CAD build for the part. Positions are in the model's coordinates, mm. A direction names the side the tool comes from. Round coordinates to 2 decimals unless told otherwise and drop trailing zeros. Order: outer loops, then holes, each group sorted by start corner. A loop starts at its lowest first (then second) coordinate and runs counter-clockwise, first axis right, second up. Notation, with made-up numbers: M -30.75,79 L 4.25,79 A27 cw 4.25,101 Z; hole C -34.5,49 d4. An arc over 180 degrees is marked long. Answer as a JSON object with one key per item and string values.
```python
from build123d import *

# Parameters (mm, degrees)
SKETCH_1_W                   = 25
SKETCH_1_H                   = 10
EXTRUDE_1_DEPTH              = 4
SKETCH_2_W                   = 7
SKETCH_2_H                   = 1
CUT_EXTRUDE_1_DEPTH          = 17.5
HOLE_WIZARD_M3_1_D           = 3.4
HOLE_WIZARD_M3_1_CSINK_D     = 6.6
HOLE_WIZARD_M3_1_CSINK_ANGLE = 90
FILLET_1_R                   = 2
CHAMFER_1_SIZE               = 0.4
CUT_EXTRUDE_2_DEPTH          = 0.4


with BuildPart() as part:
    # 草图1 → 凸台-拉伸1 (new body)
    with BuildSketch(Plane.XY):
        Rectangle(SKETCH_1_W, SKETCH_1_H)
    extrude(amount=EXTRUDE_1_DEPTH)

    # 草图2 → 切除-拉伸1 (cut, through all)
    with BuildSketch(Plane(origin=(0, 5, 0), x_dir=(1, 0, 0), z_dir=(0, 1, 0))):
        Rectangle(SKETCH_2_W, SKETCH_2_H)
    extrude(amount=-CUT_EXTRUDE_1_DEPTH, mode=Mode.SUBTRACT)

    # M3 十字槽沉头木螺钉的锥形沉头孔1 (through all)
    with Locations(Plane.XY.offset(4)):
        with Locations((7, 0)):
            hole_wizard_m3_1 = CounterSinkHole(HOLE_WIZARD_M3_1_D / 2, HOLE_WIZARD_M3_1_CSINK_D / 2, counter_sink_angle=HOLE_WIZARD_M3_1_CSINK_ANGLE)

    # 镜向1: M3 十字槽沉头木螺钉的锥形沉头孔1 across plane
    add(hole_wizard_m3_1.mirror(Plane(origin=(0, 0, 0), x_dir=(0, 0, 1), z_dir=(1, 0, 0))), mode=Mode.SUBTRACT)

    # 圆角1
    fillet_1_edges = [part.edges().sort_by_distance(p)[0] for p in [
        (12.5, -5, 2),
        (-12.5, -5, 2),
        (-12.5, 5, 2),
        (12.5, 5, 2),
    ]]
    fillet(fillet_1_edges, radius=FILLET_1_R)

    # 倒角1
    chamfer_1_edges = [part.edges().sort_by_distance(p)[0] for p in [
        (-12.5, 0, 4),
        (0, 5, 4),
        (12.5, 0, 4),
        (0, -5, 4),
        (11.914213562, 4.414213562, 4),
        (11.914213562, -4.414213562, 4),
        (-11.914213562, -4.414213562, 4),
        (-11.914213562, 4.414213562, 4),
    ]]
    chamfer(chamfer_1_edges, length=CHAMFER_1_SIZE)

    # 草图5 → 切除-拉伸2 (cut)
    with BuildSketch(Plane(origin=(0, 0, 0.5), x_dir=(-1, 0, 0), z_dir=(0, 0, -1))):
        Polygon((-3.5, -2.085786438), (-3.5, -3.5), (3.5, 3.5), (3.5, 4.914213562), align=None)
        Polygon((3.5, 0.5), (3.5, 1.914213562), (-3.414213562, -5), (-2, -5), align=None)
        Polygon((-3.5, 0.914213562), (-3.5, -0.5), (2, 5), (0.585786438, 5), align=None)
        Polygon((3.5, -2.5), (3.5, -1.085786438), (-0.414213562, -5), (1, -5), align=None)
        Polygon((-3.5, 3.914213562), (-3.5, 2.5), (-1, 5), (-2.414213562, 5), align=None)
        Polygon((3.5, -5), (3.5, -4.085786438), (2.585786438, -5), align=None)
    extrude(amount=-CUT_EXTRUDE_2_DEPTH, mode=Mode.SUBTRACT)


solid = part.part
```
Item 1: Saw through at B-B on z = 3.35. List the corners of the cut face in (x, y), and give its area (3 significant figures).
Worked answers:
{"outline": "M -12.5,-3 A2 ccw -10.5,-5 L 10.5,-5 A2 ccw 12.5,-3 L 12.5,3 A2 ccw 10.5,5 L -10.5,5 A2 ccw -12.5,3 Z; hole C -7,0 d5.3; hole C 7,0 d5.3", "area": "202 mm2"}
Item 2: Saw through at C-C on y = 0. State how many separate pieces and enclosed holes the cut face has, and give its area (3 significant figures).
Worked answers:
{"separate pieces": "3", "enclosed holes": "0", "area": "62.7 mm2"}
Item 3: Wall check: line 1 along X through (y, z) = (0, 1.4); line 2 along Y through (x, z) = (-7, 1.5); line 3 along Y through (x, z) = (-3.25, 0.6). Give the ranges that are in metal, low to high. Write a range as [from, to].
Worked answers:
{"line 1": "x = [-12.5, -8.7], [-5.3, 5.3], [8.7, 12.5]", "line 2": "y = [-5, -1.7], [1.7, 5]", "line 3": "y = [-4.34, -2.75], [-1.34, 0.25], [1.66, 3.25], [4.66, 5]"}
Item 4: Drop a flat-ended pin along its axis: pin 1 Ø3 at (x, y) = (1.5, 4) entering from -Z. Give the stop position or say it passes through.
Worked answers:
{"pin 1": "stops at z = 0.5"}
Item 5: 3-axis set-ups, long thin cutter, end or side, ignore diameter. For faces 1 (the flat face through (-2.2, -3.8, 0.7)), 2 (the flat face through (-1, -3, 0.5)), 3 (the flat face through (-9, 0, 0)): which of +Z, -Z, +X, -X, +Y, -Y reach the whole face in a straight line?
Worked answers:
{"face 1": "-Z", "face 2": "-Z, +Y, -Y", "face 3": "-Z, +X, -X, +Y, -Y"}
Item 6: Saw through at D-D on z = 1.75. List the corners of the cut face in (x, y), and give its area (3 significant figures).
Worked answers:
{"outline": "M -12.5,-3 A2 ccw -10.5,-5 L 10.5,-5 A2 ccw 12.5,-3 L 12.5,3 A2 ccw 10.5,5 L -10.5,5 A2 ccw -12.5,3 Z; hole C -7,0 d3.4; hole C 7,0 d3.4", "area": "228 mm2"}
Item 7: Two-plate mould, pull along Y, no slides. Class faces 4 (the flat face through (-0.049, 1.463, 0.697)), 5 (the cylindrical face through (11.93, 4.4, 1.83)), 6 (the flat face through (9, 0, 0)), 7 (the cylindrical face through (11.93, -4.4, 1.83)): released by +Y, released by -Y, zero draft, split by the parting line, or undercut.
Worked answers:
{"face 4": "undercut", "face 5": "released by +Y", "face 6": "zero draft", "face 7": "released by -Y"}
Item 8: Saw through at A-A on x = 7. List the corners of the cut face in (y, z), and give its area (3 significant figures).
Worked answers:
{"outline": "M -5,0 L -1.7,0 L -1.7,2.4 L -3.3,4 L -4.6,4 L -5,3.6 Z; M 1.7,0 L 5,0 L 5,3.6 L 4.6,4 L 3.3,4 L 1.7,2.4 Z", "area": "23.7 mm2"}
